Verification items for the finished model (mm, model axes). A direction names the side the tool comes from. Round coordinates to 2 decimals unless told otherwise and drop trailing zeros. Loops run counter-clockwise (first coordinate to the right, second up) from the corner with the lowest first, then second, coordinate; pieces in that order, holes last. Notation, with made-up numbers: M 70.5,88 L 122.5,88 A18 ccw 122.5,105 Z; hole C 76,-1 d4. An arc over 180 degrees is marked long. Answer as CSV lines item,"result".
```python
from build123d import *

# Parameters (mm, degrees)
PAD_DEPTH            = 9
SKETCH001_W          = 37.346859
SKETCH001_H          = 35.838272
POCKET_DEPTH         = 6
POCKET_DEPTH_BACK    = -100
SKETCH002_R          = 2.5
POCKET001_DEPTH      = 38.001
SKETCH003_R          = 2.5
POCKET002_DEPTH      = 38.001
SKETCH004_W          = 20
SKETCH004_H          = 20
POCKET003_DEPTH      = 9.001
POCKET003_DEPTH_BACK = -9.001


with BuildPart() as part:
    # Sketch → Pad (new body, symmetric)
    with BuildSketch(Plane.XY):
        Polygon((0, 0), (0, 38), (5, 38), (38, 5), (38, 0), align=None)
    extrude(amount=PAD_DEPTH, both=True)

    # Sketch001 → Pocket (cut, two sides)
    with BuildSketch(Plane.XY) as pocket_sk:
        with Locations((23.673429, 22.919136)):
            Rectangle(SKETCH001_W, SKETCH001_H)
    extrude(amount=-POCKET_DEPTH, mode=Mode.SUBTRACT)
    extrude(pocket_sk.sketch, amount=-POCKET_DEPTH_BACK, mode=Mode.SUBTRACT)

    # Sketch002 (on Face2 of Pocket) → Pocket001 (cut, through all)
    with BuildSketch(Plane.XZ):
        with Locations((15, 0)):
            Circle(SKETCH002_R)
        with Locations((30, 0)):
            Circle(SKETCH002_R)
    extrude(amount=-POCKET001_DEPTH, mode=Mode.SUBTRACT)

    # Sketch003 (on Face1 of Pocket001) → Pocket002 (cut, through all)
    with BuildSketch(Plane(origin=(0, 0, 0), x_dir=(0, -1, 0), z_dir=(-1, 0, 0))):
        with Locations((-30, 0)):
            Circle(SKETCH003_R)
        with Locations((-15, 0)):
            Circle(SKETCH003_R)
    extrude(amount=-POCKET002_DEPTH, mode=Mode.SUBTRACT)

    # Sketch004 → Pocket003 (cut, two sides)
    with BuildSketch(Plane.XY) as pocket003_sk:
        with Locations((15, 30)):
            Rectangle(SKETCH004_W, SKETCH004_H)
    extrude(amount=-POCKET003_DEPTH, mode=Mode.SUBTRACT)
    extrude(pocket003_sk.sketch, amount=-POCKET003_DEPTH_BACK, mode=Mode.SUBTRACT)


solid = part.part
```
1) Go/stop test with flat-tipped pins: pin 1 (4.5 mm diameter, centred on x = 16, y = 12, fed in from +Z); pin 2 (6 mm diameter, centred on y = 15, z = 0, fed in from +X); pin 3 (8 mm diameter, centred on x = 30, z = 0, fed in from +Y). Record where each tip stops, or that it passes through.
Here are the results:
pin 1,"stops at z = -6"
pin 2,"stops at x = 5"
pin 3,"stops at y = 5"
2) Section check C-C (z = 0). Record the cut outline in (x, y).
Here are the results:
outline,"M 0,0 L 12.5,0 L 12.5,5 L 5,5 L 5,12.5 L 0,12.5 Z; M 0,17.5 L 5,17.5 L 5,27.5 L 0,27.5 Z; M 0,32.5 L 5,32.5 L 5,38 L 0,38 Z; M 17.5,0 L 27.5,0 L 27.5,5 L 17.5,5 Z; M 32.5,0 L 38,0 L 38,5 L 32.5,5 Z"
3) Section check B-B (x = 30). Record the cut outline in (y, z).
Here are the results:
outline,"M 0,-9 L 13,-9 L 13,-6 L 5,-6 L 5,-2.5 L 0,-2.5 Z; M 0,2.5 L 5,2.5 L 5,9 L 0,9 Z"
4) Set-up check for faces 1 (the flat face through (14, 20, -7)), 2 (the flat face through (0, 19, 0)): record each of +Z, -Z, +X, -X, +Y, -Y from which the full face is reachable in a straight line by a thin tool's end or side.
Here are the results:
face 1,"+Z, -Z, +X, +Y"
face 2,"+Z, -Z, -X, +Y, -Y"
5) Section check A-A (y = 31.5). Record the cut outline in (x, z), plus the area to 3 significant figures.
Here are the results:
outline,"M 0,-9 L 5,-9 L 5,-2 L 0,-2 Z; M 0,2 L 5,2 L 5,9 L 0,9 Z"
area,"70.0 mm^2"
6) Material ranges on probe 1 along Z at (x, y) = (30, 3); probe 2 along Y at (x, z) = (26, -4.25), recorded low to high.
Here are the results:
probe 1,"z = -9 to -2.5, 2.5 to 9"
probe 2,"y = 0 to 5"
7) Section check D-D (y = 15). Record the cut outline in (x, z), plus the area to 3 significant figures.
Here are the results:
outline,"M 0,-9 L 28,-9 L 28,-6 L 5,-6 L 5,-2.5 L 0,-2.5 Z; M 0,2.5 L 5,2.5 L 5,9 L 0,9 Z"
area,"134 mm^2"
8) Draft check along Z on faces 3 (the cylindrical face through (27.5, 2.5, 0.1)), 4 (the flat face through (21, 5, 1)), 5 (the cylindrical face through (12.5, 2.5, 0.1)), 6 (the flat face through (18, 13, -6)). Enter one of: +Z half, -Z half, draft (parallel to the pull), parting line (faces both ways), or undercut.
Here are the results:
face 3,"undercut"
face 4,"draft"
face 5,"undercut"
face 6,"+Z half"
